The model under review builds one solid part; all positions refer to its coordinate system, in mm. Face numbers are marked on the shaded views. Coordinates: 2 decimals unless noted, no trailing zeros. Loops run counter-clockwise (first coordinate to the right, second up) from the corner with the lowest first, then second, coordinate; pieces in that order, holes last. Notation, with made-up numbers: M 76,3.25 L 95,3.25 A24 cw 95,39.25 Z; hole C 27.5,28 d11. An arc over 180 degrees is marked long. One line per item, written item: value.
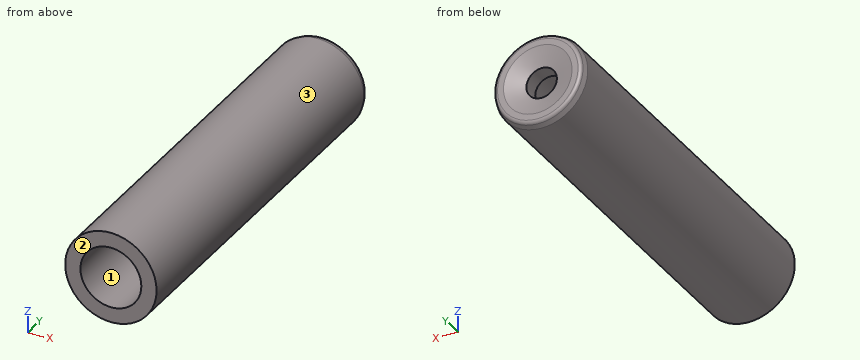
```python
from build123d import *

# Parameters (mm, degrees)
CROQUIS1_R              = 6
CROQUIS1_R_2            = 4
SALIENTE_EXTRUIR1_DEPTH = 40
CROQUIS2_R              = 4
SALIENTE_EXTRUIR2_DEPTH = 3
CROQUIS3_R              = 2
CORTAR_EXTRUIR1_DEPTH   = 40
CHAFL_N1_SIZE           = 2.5
CHAFL_N1_SIZE2          = 0.909925586
CHAFL_N2_SIZE           = 1
CHAFL_N2_SIZE2          = 0.363970234
REDONDEO1_R             = 0.5
CROQUIS4_R              = 6
CROQUIS4_R_2            = 4
SALIENTE_EXTRUIR3_DEPTH = 10


with BuildPart() as part:
    # Croquis1 → Saliente-Extruir1 (new body)
    with BuildSketch(Plane(origin=(0, 0, 0), x_dir=(1, 0, 0), z_dir=(0, 1, 0))):
        Circle(CROQUIS1_R)
        Circle(CROQUIS1_R_2, mode=Mode.SUBTRACT)
    extrude(amount=SALIENTE_EXTRUIR1_DEPTH)

    # Croquis2 → Saliente-Extruir2 (add)
    with BuildSketch(Plane(origin=(0, 37, 0), x_dir=(1, 0, 0), z_dir=(0, 1, 0))):
        Circle(CROQUIS2_R)
    extrude(amount=SALIENTE_EXTRUIR2_DEPTH)

    # Croquis3 → Cortar-Extruir1 (cut)
    with BuildSketch(Plane(origin=(0, 40, 0), x_dir=(1, 0, 0), z_dir=(0, 1, 0))):
        Circle(CROQUIS3_R)
    extrude(amount=-CORTAR_EXTRUIR1_DEPTH, mode=Mode.SUBTRACT)

    # Chaflán1
    chafl_n1_edges = [part.edges().sort_by_distance(p)[0] for p in [
        (-2, 40, 0),
    ]]
    chafl_n1_side = [part.faces().sort_by_distance(p)[0] for p in [
        (-5.830294373, 40, 0),
    ]]
    chamfer(chafl_n1_edges, length=CHAFL_N1_SIZE, length2=CHAFL_N1_SIZE2, reference=chafl_n1_side[0])

    # Chaflán2
    chafl_n2_edges = [part.edges().sort_by_distance(p)[0] for p in [
        (-6, 40, 0),
    ]]
    chafl_n2_side = [part.faces().sort_by_distance(p)[0] for p in [
        (-6, 20, 0),
    ]]
    chamfer(chafl_n2_edges, length=CHAFL_N2_SIZE, length2=CHAFL_N2_SIZE2, reference=chafl_n2_side[0])

    # Redondeo1
    redondeo1_edges = [part.edges().sort_by_distance(p)[0] for p in [
        (-5.636029766, 40, 0),
    ]]
    fillet(redondeo1_edges, radius=REDONDEO1_R)

    # Croquis4 → Saliente-Extruir3 (add)
    with BuildSketch(Plane.XZ):
        Circle(CROQUIS4_R)
        Circle(CROQUIS4_R_2, mode=Mode.SUBTRACT)
    extrude(amount=SALIENTE_EXTRUIR3_DEPTH)


solid = part.part
```
(1) Insertion check: pin 1 Ø6.5 at (x, z) = (0, 0) entering from -Y; pin 2 Ø1.5 at (x, y) = (3.5, -4) entering from -Z; pin 3 Ø6 at (x, y) = (3.5, 1.5) entering from +Z; pin 4 Ø6 at (y, z) = (0.5, -2) entering from -X. Each pin has a flat end and moves straight along its axis. Give the tip position at first contact, or say it passes through.
Checks:
pin 1: y = 37
pin 2: z = -5.33
pin 3: z = 5.98
pin 4: x = -6
(2) To check wall thickness, follow L1, parallel to Z at x = 0, y = 38.05; L2, parallel to X at y = 26, z = 0; L3, parallel to Z at x = -0.25, y = 14. State the ranges of each line that lie inside material, in increasing order. Write a range as [from, to].
Checks:
L1: [-6, -2], [2, 6]
L2: [-6, -4], [4, 6]
L3: [-5.99, -3.99], [3.99, 5.99]
(3) Add section C-C on y = 34. State the section outline as (x, z) points.
Checks:
outline: C 0,0 d12; hole C 0,0 d8
(4) Add section A-A on x = 0. State the section outline as (y, z) points, then the cut area to 3 significant figures.
Checks:
outline: M -10,-6 L 39,-6 L 39.67,-5.76 A0.5 ccw 40,-5.29 L 40,-4.5 L 39.09,-2 L 37,-2 L 37,-4 L -10,-4 Z; M -10,4 L 37,4 L 37,2 L 39.09,2 L 40,4.5 L 40,5.29 A0.5 ccw 39.67,5.76 L 39,6 L -10,6 Z
area: 209 mm^2
(5) Add section B-B on z = 0. State the section outline as (x, y) points, then the cut area to 3 significant figures.
Checks:
outline: M -6,-10 L -4,-10 L -4,37 L -2,37 L -2,39.09 L -4.5,40 L -5.29,40 A0.5 ccw -5.76,39.67 L -6,39 Z; M 2,37 L 4,37 L 4,-10 L 6,-10 L 6,39 L 5.76,39.67 A0.5 ccw 5.29,40 L 4.5,40 L 2,39.09 Z
area: 209 mm^2
(6) Draft analysis for pull direction X (two halves, no side actions). For the marked faces 1, 2 and 3, state which applies: pulls with the +X half, pulls with the -X half, needs draft (parallel to the pull), parting line crosses it, or undercut.
Checks:
face 1: undercut
face 2: needs draft
face 3: parting line crosses it
